Model file for the job. Use its own axes, mm. A direction names the side the tool comes from. Coordinates: 2 decimals unless noted, no trailing zeros. Write each loop counter-clockwise with the first axis right and the second up, starting at its lowest first coordinate (ties: lowest second). Pieces come first, ordered by that corner, then holes. Notation, with made-up numbers: M -34,82 L -24,82 A24 ccw -24,98 Z; hole C -21.5,-38.75 d11. An arc over 180 degrees is marked long. Put each result on its own line as item: value. Start each with the question number.
Q1. Which spindle directions (+Z, -Z, +X, -X, +Y, -Y) get a long thin tool onto all of the face, cutting with end or side? Do faces 1 (the flat face through (-38.961, 19.764, 0.782)), 2 (the flat face through (-29.52, 24.64, 0.78)). Say none if no direction does.
Q2. Drop a flat-ended pin along its axis: pin 1 (5.5 mm diameter, centred on x = -95.09, y = 0, fed in from +Z). Give the stop position or say it passes through.
Q3. Pull direction X, two halves, no side cores. Call faces 3 (the cylindrical face through (-13.798, 0.956, 0.782)), 4 (the flat face through (-65, 25, 0)), 5 (the flat face through (-57.44, -4.78, 0.78)), 6 (the cylindrical face through (-4.692, 1.432, 0.805)): pulls with the +X half, pulls with the -X half, needs draft (parallel to the pull), parting line crosses it, or undercut.
Q4. Drill centre lines: line 1 along Y through (x, z) = (-60, 1.1); line 2 along X through (y, z) = (5.5, 1.2); line 3 along Y through (x, z) = (-96.5, 0.35). Where is each one in solid material? Low to high.
Q5. Cut at C-C (z = 1.3). Write the cut outline in (x, y) (3 decimals), then the cut area to 3 significant figures.
Q6. Cut at A-A (x = -73). Write the cut outline in (y, z).
Q7. Cut at B-B (y = 41.5). Write the cut outline in (x, z), then the cut area to 3 significant figures.
```python
from build123d import *

# Parameters (mm, degrees)
ESQUISSE1_R        = 3.302
BOSS_EXTRU_2_DEPTH = 1.587
CONG_1_R           = 3


with BuildPart() as part:
    # Esquisse1 → Boss.-Extru.2 (new body)
    with BuildSketch(Plane(origin=(0, 0, 0), x_dir=(0, 1, 0), z_dir=(0, 0, 1))):
        with BuildLine():
            Line((-0.865912697, 10.406603399), (0, 0))
            Line((0, 0), (45.164905045, 54.107342637))
            ThreePointArc((45.164905045, 54.107342637), (46.860747383, 60.617730495), (42.915369181, 66.067044408))
            ThreePointArc((42.915369181, 66.067044408), (22.727341061, 80.577470806), (6.560094465, 99.464744063))
            ThreePointArc((6.560094465, 99.464744063), (-2.596669453, 102.535168417), (-7.857844745, 94.436164423))
            Line((-7.857844745, 94.436164423), (-1.612927072, 19.384277892))
            ThreePointArc((-1.612927072, 19.384277892), (-2.927440017, 14.754983859), (-0.865912697, 10.406603399))
        make_face()
        with Locations(Location((3.885, 15.321833395, 0), (0, 0, 270))):
            Circle(ESQUISSE1_R, mode=Mode.SUBTRACT)
        with BuildLine():
            Line((5, 22.066270538), (5, 82.747179925))
            ThreePointArc((5, 82.747179925), (19.367518455, 70.82097994), (31.370848456, 56.517836875))
            Line((31.370848456, 56.517836875), (7.827581381, 20.90633959))
            ThreePointArc((7.827581381, 20.90633959), (6.479444508, 21.646350379), (5, 22.066270538))
        make_face(mode=Mode.SUBTRACT)
        with Locations(Location((0, 95.09, 0), (0, 0, 270))):
            Circle(ESQUISSE1_R, mode=Mode.SUBTRACT)
        with Locations(Location((39.111633766, 59.160176675, 0), (0, 0, 270))):
            Circle(ESQUISSE1_R, mode=Mode.SUBTRACT)
    extrude(amount=BOSS_EXTRU_2_DEPTH)

    # Congé1
    cong_1_edges = [part.edges().sort_by_distance(p)[0] for p in [
        (0, 0, 0.7935),
    ]]
    fillet(cong_1_edges, radius=CONG_1_R)


solid = part.part
```
Computed values:
1. face 1: +Z, -Z
1. face 2: +Z, -Z, +X, +Y
2. pin 1: through
3. face 3: undercut
3. face 4: needs draft
3. face 5: undercut
3. face 6: pulls with the +X half
4. line 1: -4.99 to 5, 28.84 to 35.92, 42.31 to 46.95
4. line 2: -100.74 to -82.4, -21.96 to -18.2, -12.44 to -6.59
4. line 3: -7.76 to -2.99, 2.99 to 8.61
5. outline: M -99.465,6.56 A7.885 ccw -94.436,-7.858 L -19.384,-1.613 A6.836 ccw -10.407,-0.866 L -7.288,-0.606 A3 ccw -5.614,4.686 L -54.107,45.165 A7.885 ccw -66.067,42.915 A104 cw Z; hole C -95.09,0 d6.604; hole M -82.747,5 L -22.066,5 A6.836 cw -20.906,7.828 L -56.518,31.371 A104 ccw Z; hole C -59.16,39.112 d6.604; hole C -15.322,3.885 d6.604
5. area: 1,930 mm2
6. outline: M -6.07,0 L 5,0 L 5,1.59 L -6.07,1.59 Z; M 17.11,0 L 31.99,0 L 31.99,1.59 L 17.11,1.59 Z
7. outline: M -66.86,0 L -61.44,0 L -61.44,1.59 L -66.86,1.59 Z; M -56.88,0 L -49.72,0 L -49.72,1.59 L -56.88,1.59 Z
7. area: 20.0 mm2
